```python
from build123d import *

# Parameters (mm, degrees)
SKETCH1_R           = 1.5
BOSS_EXTRUDE1_DEPTH = 3
FILLET1_R           = 10
FILLET2_START       = -1
FILLET2_DEPTH       = 5
FILLET3_RADIUS      = 5
FILLET3_LENGTH      = 3


with BuildPart() as part:
    # Sketch1 → Boss-Extrude1 (new body)
    with BuildSketch(Plane.XY):
        with BuildLine():
            Line((-40.5, 20), (-40.5, -10))
            Line((-40.5, -10), (-30.5, -10))
            Line((-30.5, -10), (-30.5, 12))
            Line((-30.5, 12), (10.5, 12))
            Line((10.5, 12), (10.5, -10))
            Line((10.5, -10), (20, -10))
            add(Edge.make_bspline(
                [(118.084820575, 20.381332685), (20, 39.436163422), (20, -10)],
                knots=[0, 0, 0, 1, 1, 1], degree=2))
            ThreePointArc((118.084820575, 20.381332685), (124.650748454, 23.164097275), (121.756088913, 29.681468971))
            ThreePointArc((121.756088913, 29.681468971), (39.600152782, 42.067632947), (-40.5, 20))
        make_face()
        with Locations((-34.5, -5)):
            Circle(SKETCH1_R, mode=Mode.SUBTRACT)
        with Locations((-34.5, 5)):
            Circle(SKETCH1_R, mode=Mode.SUBTRACT)
        with Locations((14.5, 5)):
            Circle(SKETCH1_R, mode=Mode.SUBTRACT)
        with Locations((14.5, -5)):
            Circle(SKETCH1_R, mode=Mode.SUBTRACT)
    extrude(amount=BOSS_EXTRUDE1_DEPTH)

    # Fillet1
    fillet1_edges = [part.edges().sort_by_distance(p)[0] for p in [
        (-40.5, 20, 1.5),
    ]]
    fillet(fillet1_edges, radius=FILLET1_R)

    # Fillet2: read off the stored shape, not the designer's step
    # Fillet2 outline → Fillet2 (cut)
    with BuildSketch(Plane.XY.offset(FILLET2_START)):
        with BuildLine():
            add(Edge.make_bspline(
                [(20, -10), (20, -7.730924257), (20.206638038, -5.606140409)],
                knots=[0, 0, 0, 0.045899107, 0.045899107, 0.045899107], degree=2))
            add(Edge.make_bspline(
                [(20.206638038, -5.606140409), (19.985493057, -7.880093874), (18.329539971, -9.999999869), (15.36474074, -10)],
                knots=[0, 0, 0, 0, 0.487277065, 0.487277065, 0.487277065, 0.487277065], degree=3, weights=[1, 0.690889052, 0.53240078, 0.524535183]))
            Line((15.36474074, -10), (20, -10))
        make_face()
        with BuildLine():
            Line((10.5, -10), (15.36474074, -10))
            add(Edge.make_bspline(
                [(15.36474074, -10), (12.147576418, -10.000000142), (10.5, -7.59675874), (10.5, -5.135259475)],
                knots=[0.487277065, 0.487277065, 0.487277065, 0.487277065, 1, 1, 1, 1], degree=3, weights=[0.524535183, 0.51625884, 0.674747113, 1]))
            Line((10.5, -5.135259475), (10.5, -10))
        make_face()
    extrude(amount=FILLET2_DEPTH, mode=Mode.SUBTRACT)

    # Fillet3: full round fillet: the end face becomes a half cylinder, R = half its width
    fillet3_face = Plane((-35.5, -10, 1.5), x_dir=(0, 0, 1), z_dir=(0, -1, 0))  # on the end face: x along it, z out of the body
    fillet3_slab = fillet3_face.offset(-FILLET3_RADIUS / 2) * Box(FILLET3_LENGTH, 2 * FILLET3_RADIUS, FILLET3_RADIUS, mode=Mode.PRIVATE)  # the body's end, R deep
    fillet3_round = Plane((-35.5, -5, 1.5), x_dir=(0, -1, 0), z_dir=(0, 0, 1)) * Cylinder(FILLET3_RADIUS, FILLET3_LENGTH, mode=Mode.PRIVATE)  # its axis R under the face
    add(fillet3_slab - fillet3_round, mode=Mode.SUBTRACT)


solid = part.part
```
Geometry: final body of the model. Coordinates: model frame, mm. A direction names the side the tool comes from. Coordinates: 2 decimals unless noted, no trailing zeros. Loops run counter-clockwise (first coordinate to the right, second up) from the corner with the lowest first, then second, coordinate; pieces in that order, holes last. Notation, with made-up numbers: (73.25, 36.25) -> (120.25, 36.25) arc R25 cw to (120.25, 53.25) -> close; hole circle Ø9 at (23.5, 2). An arc over 180 degrees is marked (long way). Use a Markdown table: item, result. Add a question column.
(1) Access query for faces 4 (the flat face through (10.5, 4, 1)), 5 (the flat face through (23, 22, 0)). Directions: +Z, -Z, +X, -X, +Y, -Y. A direction counts if a zero-diameter tool reaches every point of the face in a straight line with its end or side. Return the directions, or none.
(2) Mould query, pull axis Y, two halves, no side actions, for faces 1 (the cylindrical face through (124.61, 23.06, 1.48)), 2 (the cylindrical face through (43.897, 42.278, 1.479)), 3 (the cylindrical face through (13, 5, 1)). Classes: pulls with the +Y half, pulls with the -Y half, needs draft (parallel to the pull), parting line crosses it, or undercut.
(3) Pin query (flat end, axial travel): pin 1 Ø1.8 at (x, y) = (-34.5, 5) entering from +Z; pin 2 Ø1.5 at (x, z) = (79.5, 1.5) entering from -Y. Return the tip coordinate at first contact, or that it passes through.
(4) Section query B-B, the plane x = 120. Return loops of the section in (y, z).
(5) Line query: line 1 along Y through (x, z) = (-34.5, 1.5); line 2 along Y through (x, z) = (14.5, 0.95); line 3 along X through (y, z) = (-1, 0.35). Output: solid intervals per line, ascending.
(6) Section query A-A, the plane y = 5. State how many separate pieces and enclosed holes the cut face has, plus the area to 3 significant figures.
(7) Section query D-D, the plane y = 37. Return loops of the section in (x, z), plus the area to 3 significant figures.
Answer:
| question | item | result |
|---|---|---|
| 1 | face 4 | +Z, -Z, -Y |
| 1 | face 5 | -Z, +X, -X, +Y, -Y |
| 2 | face 1 | parting line crosses it |
| 2 | face 2 | pulls with the +Y half |
| 2 | face 3 | undercut |
| 3 | pin 1 | passes through |
| 3 | pin 2 | stops at y = 25.42 |
| 4 | outline | (20, 0) -> (30.33, 0) -> (30.33, 3) -> (20, 3) -> close |
| 5 | line 1 | y = -9.9 to -6.5, -3.5 to 3.5, 6.5 to 22.98 |
| 5 | line 2 | y = -9.92 to -6.5, -3.5 to 3.5, 6.5 to 38.97 |
| 5 | line 3 | x = -40.5 to -30.5, 10.5 to 20.93 |
| 6 | separate pieces | 4 |
| 6 | enclosed holes | 0 |
| 6 | area | 49.2 mm^2 |
| 7 | outline | (5.26, 0) -> (97.77, 0) -> (97.77, 3) -> (5.26, 3) -> close |
| 7 | area | 278 mm^2 |
